from build123d import *

# Parameters (mm, degrees)
SKETCH1_W           = 280
SKETCH1_H           = 70
BOSS_EXTRUDE1_DEPTH = 7
FILLET1_R           = 6
SKETCH2_R           = 15
SKETCH2_R_2         = 4
CUT_EXTRUDE1_DEPTH  = 10
BOSS_EXTRUDE2_START = 2
SKETCH3_R           = 20
SKETCH3_R_2         = 15
BOSS_EXTRUDE2_DEPTH = 2
CUT_EXTRUDE2_DEPTH  = 3


with BuildPart() as part:
    # Sketch1 → Boss-Extrude1 (new body)
    with BuildSketch(Plane.XY):
        Rectangle(SKETCH1_W, SKETCH1_H)
    extrude(amount=BOSS_EXTRUDE1_DEPTH)

    # Fillet1
    fillet1_edges = [part.edges().sort_by_distance(p)[0] for p in [
        (140, -35, 3.5),
        (-140, -35, 3.5),
        (-140, 35, 3.5),
        (140, 35, 3.5),
    ]]
    fillet(fillet1_edges, radius=FILLET1_R)

    # Sketch2 → Cut-Extrude1 (cut)
    with BuildSketch(Plane(origin=(0, 0, 0), x_dir=(-1, 0, 0), z_dir=(0, 0, -1))):
        with Locations((-107.5, 0)):
            Circle(SKETCH2_R)
        with Locations((107.5, 0)):
            Circle(SKETCH2_R)
        with Locations((130, 25)):
            Circle(SKETCH2_R_2)
        with Locations((65, 25)):
            Circle(SKETCH2_R_2)
        with Locations((-65, 25)):
            Circle(SKETCH2_R_2)
        with Locations((-130, 25)):
            Circle(SKETCH2_R_2)
        with Locations(Location((-130, -25, 0), (0, 0, 180))):
            Circle(SKETCH2_R_2)
        with Locations(Location((-65, -25, 0), (0, 0, 180))):
            Circle(SKETCH2_R_2)
        with Locations(Location((65, -25, 0), (0, 0, 180))):
            Circle(SKETCH2_R_2)
        with Locations(Location((130, -25, 0), (0, 0, 180))):
            Circle(SKETCH2_R_2)
        with BuildLine():
            Line((-2.5, 2.5), (-2.5, 20.383453672))
            ThreePointArc((-2.5, 20.383453672), (0, 30.25), (2.5, 20.383453672))
            Line((2.5, 20.383453672), (2.5, 2.5))
            ThreePointArc((2.5, 2.5), (0, 0), (-2.5, 2.5))
        make_face()
    extrude(amount=-CUT_EXTRUDE1_DEPTH, mode=Mode.SUBTRACT)

    # Sketch3 → Boss-Extrude2 (add)
    # profile 1 of 2: a face of its own
    with BuildSketch(Plane(origin=(0, 0, 0), x_dir=(-1, 0, 0), z_dir=(0, 0, -1)).offset(BOSS_EXTRUDE2_START)):
        with Locations(Location((-107.5, 0, 0), (0, 0, 180))):
            Circle(SKETCH3_R)
        with Locations((-107.5, 0)):
            Circle(SKETCH3_R_2, mode=Mode.SUBTRACT)
    # profile 2 of 2: a face of its own
    with BuildSketch(Plane(origin=(0, 0, 0), x_dir=(-1, 0, 0), z_dir=(0, 0, -1)).offset(BOSS_EXTRUDE2_START)):
        with Locations(Location((107.5, 0, 0), (0, 0, 180))):
            Circle(SKETCH3_R)
        with Locations((107.5, 0)):
            Circle(SKETCH3_R_2, mode=Mode.SUBTRACT)
    extrude(amount=-BOSS_EXTRUDE2_DEPTH)

    # Sketch4 → Cut-Extrude2 (cut)
    with BuildSketch(Plane(origin=(0, 0, 2), x_dir=(-1, 0, 0), z_dir=(0, 0, -1))):
        with BuildLine():
            Line((0, 25), (-5.25, 25))
            Line((-5.25, 25), (-5.25, 2.5))
            ThreePointArc((-5.25, 2.5), (0, -2.75), (5.25, 2.5))
            Line((5.25, 2.5), (5.25, 25))
            Line((5.25, 25), (0, 25))
        make_face()
    extrude(amount=-CUT_EXTRUDE2_DEPTH, mode=Mode.SUBTRACT)


solid = part.part
Model file for the job. Use its own axes, mm. A direction names the side the tool comes from. Coordinates: 2 decimals unless noted, no trailing zeros. Write each loop counter-clockwise with the first axis right and the second up, starting at its lowest first coordinate (ties: lowest second). Pieces come first, ordered by that corner, then holes. Notation, with made-up numbers: (17.25, 7) -> (69.25, 7) arc R11 ccw to (69.25, 14) -> close; hole circle Ø1 at (24, 6). An arc over 180 degrees is marked (long way). One line per item, written item: value. Start each with the question number.
1) Slice it at B-B on z = 3.5. Count the separate pieces of the cut face and the enclosed holes in it, then the cut area to 3 significant figures.
2) Pull direction X, two halves, no side cores. Call faces 1 (the face through (-61.185, -26.201, 3.451)), 2 (the face through (-105, -15, -2)), 3 (the face through (0.12, -2.75, 3.48)), 4 (the face through (140, 0, 3)): +X half, -X half, draft (parallel to the pull), parting line (faces both ways), or undercut.
3) Slice it at C-C on y = -25. Write the cut outline in (x, z), then the cut area to 3 significant figures.
4) Which spindle directions (+Z, -Z, +X, -X, +Y, -Y) get a long thin tool onto all of the face, cutting with end or side? Do faces 5 (the face through (87.52, -0.88, -1.01)), 6 (the face through (138.289, 33.196, 3.549)), 7 (the face through (4, 8, 2)). Say none if no direction does.
5) Slice it at D-D on x = 107.5. Write the cut outline in (y, z).
6) Flat gauge pins, fed straight in: pin 1 Ø6.5 at (x, y) = (65, 25) entering from -Z; pin 2 Ø13 at (x, y) = (-65, -25) entering from +Z; pin 3 Ø10.5 at (x, y) = (65, -25) entering from -Z. Where does each tip first touch, or does it go through?
7) Slice it at A-A on x = -130. Write the cut outline in (y, z), then the cut area to 3 significant figures.
8) Probe probe 1 along Y at (x, z) = (-130, 1.5); probe 2 along X at (y, z) = (0.5, 5.5); probe 3 along X at (y, z) = (-3, 4). List the from-to ranges inside material, lowest first.
Answers follow:
1. separate pieces: 1
1. enclosed holes: 11
1. area: 17,400 mm2
2. face 1: undercut
2. face 2: draft
2. face 3: undercut
2. face 4: +X half
3. outline: (-140, 0) -> (-134, 0) -> (-134, 7) -> (-140, 7) -> close; (-126, 0) -> (-69, 0) -> (-69, 7) -> (-126, 7) -> close; (-61, 0) -> (61, 0) -> (61, 7) -> (-61, 7) -> close; (69, 0) -> (126, 0) -> (126, 7) -> (69, 7) -> close; (134, 0) -> (140, 0) -> (140, 7) -> (134, 7) -> close
3. area: 1,740 mm2
4. face 5: -Z
4. face 6: +Z, -Z, +X, +Y
4. face 7: none
5. outline: (-35, 0) -> (-20, 0) -> (-20, -2) -> (-15, -2) -> (-15, 7) -> (-35, 7) -> close; (15, -2) -> (20, -2) -> (20, 0) -> (35, 0) -> (35, 7) -> (15, 7) -> close
6. pin 1: through
6. pin 2: z = 7
6. pin 3: z = 0
7. outline: (-35, 0) -> (-29, 0) -> (-29, 7) -> (-35, 7) -> close; (-21, 0) -> (21, 0) -> (21, 7) -> (-21, 7) -> close; (29, 0) -> (35, 0) -> (35, 7) -> (29, 7) -> close
7. area: 378 mm2
8. probe 1: -35 to -29, -21 to 21, 29 to 35
8. probe 2: -140 to -122.49, -92.51 to -1.5, 1.5 to 92.51, 122.49 to 140
8. probe 3: -140 to -122.2, -92.8 to 92.8, 122.2 to 140
